```python
from build123d import *

# Parameters (mm, degrees)
F0_R     = 3.175
F0_R_2   = 2.0955
F1_DEPTH = 6.35
F5_D     = 2.2606
F5_DEPTH = 5.08
F5_START = 0.1014065
F5_TIP   = 0.6791527577


with BuildPart() as f1:
    # F0 (on Top) → F1 (new body)
    with BuildSketch(Plane.XY):
        with BuildLine():
            ThreePointArc((-25.4, -6.35), (-20.9098719395, -4.4901280605), (-19.05, 0))
            ThreePointArc((-19.05, 0), (-20.9098719395, 4.4901280605), (-25.4, 6.35))
            ThreePointArc((-25.4, 6.35), (-31.75, 0), (-25.4, -6.35))
        make_face()
        with Locations((-25.4, 0)):
            Circle(F0_R, mode=Mode.SUBTRACT)
        with BuildLine():
            ThreePointArc((-25.4, 6.35), (-20.9098719395, 4.4901280605), (-19.05, 0))
            ThreePointArc((-19.05, 0), (-20.9098719395, -4.4901280605), (-25.4, -6.35))
            Line((-25.4, -6.35), (25.4, -6.35))
            ThreePointArc((25.4, -6.35), (19.05, 0), (25.4, 6.35))
            Line((25.4, 6.35), (12.7, 6.35))
            ThreePointArc((12.7, 6.35), (8.2098719395, 8.2098719395), (6.35, 12.7))
            Line((6.35, 12.7), (6.35, 19.05))
            ThreePointArc((6.35, 19.05), (0, 12.7), (-6.35, 19.05))
            Line((-6.35, 19.05), (-6.35, 12.7))
            ThreePointArc((-6.35, 12.7), (-8.2098719395, 8.2098719395), (-12.7, 6.35))
            Line((-12.7, 6.35), (-25.4, 6.35))
        make_face()
        Circle(F0_R, mode=Mode.SUBTRACT)
        with BuildLine():
            ThreePointArc((25.4, 6.35), (19.05, 0), (25.4, -6.35))
            ThreePointArc((25.4, -6.35), (29.8901280605, -4.4901280605), (31.75, 0))
            ThreePointArc((31.75, 0), (29.8901280605, 4.4901280605), (25.4, 6.35))
        make_face()
        with Locations((25.4, 0)):
            Circle(F0_R, mode=Mode.SUBTRACT)
        with BuildLine():
            ThreePointArc((6.35, 19.05), (0, 25.4), (-6.35, 19.05))
            ThreePointArc((-6.35, 19.05), (0, 12.7), (6.35, 19.05))
        make_face()
        with Locations((0, 19.05)):
            Circle(F0_R_2, mode=Mode.SUBTRACT)
    extrude(amount=F1_DEPTH)

    # F5
    # its depths count from where the whole tool has entered the part; down to there all is cleared
    with Locations(Plane(origin=(0, 25.4, 0), x_dir=(1, 0, 0), z_dir=(0, 1, 0)).offset(-F5_START)):
        with Locations((0, -3.175)):
            Hole(F5_D / 2, depth=F5_DEPTH)
            with Locations((0, 0, -(F5_DEPTH + F5_TIP / 2))):  # 118° drill point
                Cone(0, F5_D / 2, F5_TIP, mode=Mode.SUBTRACT)


solid = f1.part
```
Read the model definition and answer for the solid it produces. Units are mm, in the model's axes. A direction names the side the tool comes from. Round coordinates to 2 decimals unless told otherwise and drop trailing zeros. Write each loop counter-clockwise with the first axis right and the second up, starting at its lowest first coordinate (ties: lowest second). Pieces come first, ordered by that corner, then holes. Notation, with made-up numbers: (-39.5, 46.5) - (17.5, 46.5) arc R16 cw to (17.5, 68.5) - close; hole circle Ø8 at (59.5, 74). An arc over 180 degrees is marked (long way). Use CSV: the item, a comma, the result in double quotes.
Q1. Find section C-C, the plane y = 1. Write down the section's boundary in (x, z), then the cut area to 3 significant figures.
Values:
outline,"(-31.67, 0) - (-28.41, 0) - (-28.41, 6.35) - (-31.67, 6.35) - close; (-22.39, 0) - (-3.01, 0) - (-3.01, 6.35) - (-22.39, 6.35) - close; (3.01, 0) - (22.39, 0) - (22.39, 6.35) - (3.01, 6.35) - close; (28.41, 0) - (31.67, 0) - (31.67, 6.35) - (28.41, 6.35) - close"
area,"287 mm²"
Q2. Each of these flat-tipped pins is pushed along its axis until it touches: pin 1 Ø4 at (x, y) = (-16, 9.5) entering from -Z; pin 2 Ø1 at (y, z) = (-1.5, 2.5) entering from -X; pin 3 Ø3 at (x, z) = (-17.5, 2.5) entering from +Y; pin 4 Ø1.5 at (y, z) = (14, 5) entering from -X. Where does it stop, or does it pass through?
Values:
pin 1,"passes through"
pin 2,"stops at x = -31.67"
pin 3,"stops at y = 6.35"
pin 4,"stops at x = -6.35"
Q3. A tool of negligible diameter and unlimited length cuts with its end or side. For faces 4 (the flat face through (-19, 6.35, 3)), 5 (the flat face through (19, 6.35, 3)), 6 (the flat face through (0, -6.35, 3)), from which of +Z, -Z, +X, -X, +Y, -Y can it reach the whole face along a straight path? Write none if from no direction.
Values:
face 4,"+Z, -Z, -X, +Y"
face 5,"+Z, -Z, +X, +Y"
face 6,"+Z, -Z, +X, -X, -Y"
Q4. Find section A-A, the plane x = 0. Count the separate pieces of the cut face and the enclosed holes in it, then the cut area to 3 significant figures.
Values:
separate pieces,"4"
enclosed holes,"0"
area,"125 mm²"
Q5. Determine the mould class of faces 1 (the cylindrical face through (-31.75, 0.14, 3.13)), 2 (the flat face through (0, 6, 0)), 3 (the cylindrical face through (1.13, 23.08, 3.13)) for opening direction Z: +Z half, -Z half, draft (parallel to the pull), parting line (faces both ways), or undercut.
Values:
face 1,"draft"
face 2,"-Z half"
face 3,"undercut"
Q6. Straight lines are drawn through the part: line 1 along Z through (x, y) = (0, 24); line 2 along Y through (x, z) = (25.4, 3.5) (3 decimals); line 3 along Y through (x, z) = (20.5, 3). For each, find the intervals that lie inside material, in ascending order.
Values:
line 1,"z = 0 to 2.04, 4.31 to 6.35"
line 2,"y = -6.35 to -3.175, 3.175 to 6.35"
line 3,"y = -6.35 to 6.35"
Q7. Find section D-D, the plane y = 14. Write down the section's boundary in (x, z).
Values:
outline,"(-6.35, 0) - (6.35, 0) - (6.35, 6.35) - (-6.35, 6.35) - close"
